```python
from build123d import *

# Parameters (mm, degrees)
F0_W     = 151.401668787
F0_H     = 82.2127312422
F1_DEPTH = 177.8


with BuildPart() as f1:
    # F0 (on Top) → F1 (new body)
    with BuildSketch(Plane.XY):
        Polygon((0, 74.6833533049), (-75.7008343935, 35.0014641881), (75.7008343935, 35.0014641881), align=None)
        with Locations((0, -6.104901433)):
            Rectangle(F0_W, F0_H)
    extrude(amount=F1_DEPTH)


solid = f1.part
```
Geometry check sheet. Reference: the model listing, model coordinates, mm. Coordinates: 2 decimals unless noted, no trailing zeros. Loops run counter-clockwise (first coordinate to the right, second up) from the corner with the lowest first, then second, coordinate; pieces in that order, holes last.
Item 1: Sectioned sample at A-A, the plane z = 27.5. Record the boundary of the cut face in (x, y).
Item 2: Thickness scan on line 1 (Y direction, x = -11, z = 143); line 2 (Y direction, x = 14, z = 115); line 3 (X direction, y = 43, z = 120.5). Record the ranges inside material, lowest first.
Item 3: Sectioned sample at C-C, the plane x = -40. Record the boundary of the cut face in (y, z), then the cut area to 3 significant figures.
Item 4: Sectioned sample at B-B, the plane y = 45. Record the boundary of the cut face in (x, z).
Item 5: Go/stop test with a flat-tipped pin: pin 1 Ø4 at (x, z) = (37, 148) entering from +Y. Record where the tip stops, or that it passes through.
Check result:
1. outline: (-75.7, -47.21) - (75.7, -47.21) - (75.7, 35) - (0, 74.68) - (-75.7, 35) - close
2. line 1: y = -47.21 to 68.92
2. line 2: y = -47.21 to 67.34
2. line 3: x = -60.44 to 60.44
3. outline: (-47.21, 0) - (53.72, 0) - (53.72, 177.8) - (-47.21, 177.8) - close
3. area: 17,900 mm2
4. outline: (-56.63, 0) - (56.63, 0) - (56.63, 177.8) - (-56.63, 177.8) - close
5. pin 1: stops at y = 56.34
